```python
from build123d import *

# Parameters (mm, degrees)
SKETCH2_W           = 37.77
SKETCH2_H           = 5.5
BOSS_EXTRUDE1_DEPTH = 4.3


with BuildPart() as part:
    # Sketch2 → Boss-Extrude1 (new body)
    with BuildSketch(Plane.XY):
        with BuildLine():
            Line((-58.61, 69.65), (-73.61, 69.65))
            Line((-73.61, 69.65), (-73.61, 64.95))
            Line((-73.61, 64.95), (-80.7, 64.95))
            Line((-80.7, 64.95), (-80.7, 26.35))
            Line((-80.7, 26.35), (-80.318, 25.95))
            Line((-80.318, 25.95), (-68.2, 25.95))
            Line((-68.2, 25.95), (-68.2, 21.65))
            Line((-68.2, 21.65), (-80.7, 21.65))
            Line((-80.7, 21.65), (-80.7, 12.05))
            Line((-80.7, 12.05), (-85, 12.05))
            Line((-85, 12.05), (-85, -7.95))
            Line((-85, -7.95), (-80.7, -7.95))
            Line((-80.7, -7.95), (-80.7, -17.35))
            Line((-80.7, -17.35), (-56.729583067, -17.35))
            Line((-56.729583067, -17.35), (-56.729583067, -22.85))
            Line((-56.729583067, -22.85), (-80.7, -22.85))
            Line((-80.7, -22.85), (-80.7, -69.65))
            Line((-80.7, -69.65), (80.7, -69.65))
            Line((80.7, -69.65), (80.7, -22.85))
            Line((80.7, -22.85), (17.2, -22.85))
            Line((17.2, -22.85), (17.2, -17.35))
            Line((17.2, -17.35), (80.7, -17.35))
            Line((80.7, -17.35), (80.7, -7.95))
            Line((80.7, -7.95), (85, -7.95))
            Line((85, -7.95), (85, 12.05))
            Line((85, 12.05), (80.7, 12.05))
            Line((80.7, 12.05), (80.7, 21.65))
            Line((80.7, 21.65), (80.282, 21.65))
            Line((80.282, 21.65), (75.4, 21.65))
            Line((75.4, 21.65), (75.4, -1.15))
            ThreePointArc((75.4, -1.15), (72.471067812, -8.221067812), (65.4, -11.15))
            Line((65.4, -11.15), (-24.6, -11.15))
            ThreePointArc((-24.6, -11.15), (-31.671067812, -8.221067812), (-34.6, -1.15))
            Line((-34.6, -1.15), (-34.6, 33.85))
            ThreePointArc((-34.6, 33.85), (-31.671067812, 40.921067812), (-24.6, 43.85))
            Line((-24.6, 43.85), (65.4, 43.85))
            ThreePointArc((65.4, 43.85), (72.471067812, 40.921067812), (75.4, 33.85))
            Line((75.4, 33.85), (75.4, 25.95))
            Line((75.4, 25.95), (79.9, 25.95))
            Line((79.9, 25.95), (80.7, 25.95))
            Line((80.7, 25.95), (80.7, 64.95))
            Line((80.7, 64.95), (73.59, 64.95))
            Line((73.59, 64.95), (73.59, 69.65))
            Line((73.59, 69.65), (58.59, 69.65))
            Line((58.59, 69.65), (58.59, 64.95))
            Line((58.59, 64.95), (47.15, 64.95))
            Line((47.15, 64.95), (47.15, 69.65))
            Line((47.15, 69.65), (32.15, 69.65))
            Line((32.15, 69.65), (32.15, 64.95))
            Line((32.15, 64.95), (20.71, 64.95))
            Line((20.71, 64.95), (20.71, 69.65))
            Line((20.71, 69.65), (5.71, 69.65))
            Line((5.71, 69.65), (5.71, 64.95))
            Line((5.71, 64.95), (-5.73, 64.95))
            Line((-5.73, 64.95), (-5.73, 69.65))
            Line((-5.73, 69.65), (-20.73, 69.65))
            Line((-20.73, 69.65), (-20.73, 64.95))
            Line((-20.73, 64.95), (-32.17, 64.95))
            Line((-32.17, 64.95), (-32.17, 69.65))
            Line((-32.17, 69.65), (-47.17, 69.65))
            Line((-47.17, 69.65), (-47.17, 64.95))
            Line((-47.17, 64.95), (-58.61, 64.95))
            Line((-58.61, 64.95), (-58.61, 69.65))
        make_face()
        with Locations((-16.933, -20.1)):
            Rectangle(SKETCH2_W, SKETCH2_H, mode=Mode.SUBTRACT)
    extrude(amount=BOSS_EXTRUDE1_DEPTH)


solid = part.part
```
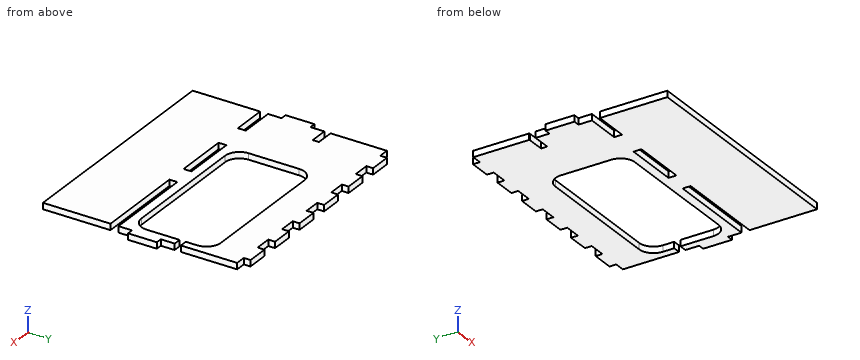
The model under review builds one solid part; all positions refer to its coordinate system, in mm. Coordinates: 2 decimals unless noted, no trailing zeros. Write each loop counter-clockwise with the first axis right and the second up, starting at its lowest first coordinate (ties: lowest second). Pieces come first, ordered by that corner, then holes. Notation, with made-up numbers: (7, 16) -> (34, 16) arc R32 cw to (34, 52) -> close; hole circle Ø4 at (14, 30.25). An arc over 180 degrees is marked (long way). One line per item, written item: value. Start each with the question number.
Q1. Add section B-B, the plane x = -15. Give the boundary of the cut face in (y, z), then the cut area to 3 significant figures.
Q2. Add section D-D, the plane y = -31.5. Give the boundary of the cut face in (x, z).
Q3. Add section C-C, the plane y = 8. Give the boundary of the cut face in (x, z).
Q4. To check wall thickness, follow probe 1 along Y at (x, z) = (-0.5, 1.2); probe 2 along Y at (x, z) = (-76.5, 2); probe 3 along Y at (x, z) = (4, 2.9). State the ranges of each line that lie inside material, in increasing order.
Q5. Clearance check with flat-ended pins moving along their axes: P1, Ø1, axis at x = 65, y = -22, coming from the -Z side; P2, Ø2, axis at y = 66, z = 2, coming from the -X side; P3, Ø1.3, axis at y = 42.5, z = 2.5, coming from the +X side; P4, Ø2, axis at x = 27.5, z = 2, coming from the +Y side. State where each tip first meets the part, or that it passes through.
Q6. Add section A-A, the plane y = 29.5. Give the boundary of the cut face in (x, z).
Response:
1. outline: (-69.65, 0) -> (-22.85, 0) -> (-22.85, 4.3) -> (-69.65, 4.3) -> close; (-17.35, 0) -> (-11.15, 0) -> (-11.15, 4.3) -> (-17.35, 4.3) -> close; (43.85, 0) -> (69.65, 0) -> (69.65, 4.3) -> (43.85, 4.3) -> close
1. area: 339 mm²
2. outline: (-80.7, 0) -> (80.7, 0) -> (80.7, 4.3) -> (-80.7, 4.3) -> close
3. outline: (-85, 0) -> (-34.6, 0) -> (-34.6, 4.3) -> (-85, 4.3) -> close; (75.4, 0) -> (85, 0) -> (85, 4.3) -> (75.4, 4.3) -> close
4. probe 1: -69.65 to -22.85, -17.35 to -11.15, 43.85 to 64.95
4. probe 2: -69.65 to -22.85, -17.35 to 21.65, 25.95 to 64.95
4. probe 3: -69.65 to -11.15, 43.85 to 64.95
5. P1: through
5. P2: x = -73.61
5. P3: x = 80.7
5. P4: y = 64.95
6. outline: (-80.7, 0) -> (-34.6, 0) -> (-34.6, 4.3) -> (-80.7, 4.3) -> close; (75.4, 0) -> (80.7, 0) -> (80.7, 4.3) -> (75.4, 4.3) -> close
